```python
from build123d import *

# Parameters (mm, degrees)
SKETCH_1_R          = 102
EXTRUDE_1_DEPTH     = 12
SKETCH_2_R          = 69
EXTRUDE_2_DEPTH     = 3
SKETCH_3_R          = 63.5
EXTRUDE_3_DEPTH     = 1
SKETCH_4_R          = 55
CUT_EXTRUDE_1_DEPTH = 146.134420452
CUT_EXTRUDE_START   = -8
SKETCH_5_R          = 82
SKETCH_5_R_2        = 69
CUT_EXTRUDE_2_DEPTH = 4
SKETCH_6_R          = 4
CUT_EXTRUDE_3_DEPTH = 8
SKETCH_7_R          = 5
CUT_EXTRUDE_4_DEPTH = 146.134420452
CHAMFER_1_SIZE      = 0.5


with BuildPart() as part:
    # 草图1 → 凸台-拉伸1 (new body)
    with BuildSketch(Plane.XY):
        Circle(SKETCH_1_R)
    extrude(amount=EXTRUDE_1_DEPTH)

    # 草图2 → 凸台-拉伸2 (add)
    with BuildSketch(Plane.XY.offset(12)):
        Circle(SKETCH_2_R)
    extrude(amount=EXTRUDE_2_DEPTH)

    # 草图3 → 凸台-拉伸3 (add)
    with BuildSketch(Plane.XY.offset(15)):
        Circle(SKETCH_3_R)
    extrude(amount=EXTRUDE_3_DEPTH)

    # 草图4 → 切除-拉伸1 (cut, through all)
    with BuildSketch(Plane.XY.offset(16)):
        Circle(SKETCH_4_R)
    extrude(amount=-CUT_EXTRUDE_1_DEPTH, mode=Mode.SUBTRACT)

    # 草图5 → 切除-拉伸2 (cut)
    with BuildSketch(Plane.XY.offset(16).offset(CUT_EXTRUDE_START)):
        Circle(SKETCH_5_R)
        Circle(SKETCH_5_R_2, mode=Mode.SUBTRACT)
    extrude(amount=CUT_EXTRUDE_2_DEPTH, mode=Mode.SUBTRACT)

    # 草图6 → 切除-拉伸3 (cut)
    with BuildSketch(Plane.XY):
        with Locations(Location((-51.265241636, 51.265241636, 0), (0, 0, 286.819656348))):
            Circle(SKETCH_6_R)
        with Locations(Location((51.265241636, 51.265241636, 0), (0, 0, 180))):
            Circle(SKETCH_6_R)
        with Locations(Location((51.265241636, -51.265241636, 0), (0, 0, 163.180343652))):
            Circle(SKETCH_6_R)
        with Locations(Location((-51.265241636, -51.265241636, 0), (0, 0, 180))):
            Circle(SKETCH_6_R)
    extrude(amount=CUT_EXTRUDE_3_DEPTH, mode=Mode.SUBTRACT)

    # 草图7 → 切除-拉伸4 (cut, through all)
    with BuildSketch(Plane(origin=(0, 0, 0), x_dir=(-1, 0, 0), z_dir=(0, 0, -1))):
        with Locations((-77.942286341, 45)):
            Circle(SKETCH_7_R)
        with Locations((0, 90)):
            Circle(SKETCH_7_R)
        with Locations((77.942286341, 45)):
            Circle(SKETCH_7_R)
        with Locations((77.942286341, -45)):
            Circle(SKETCH_7_R)
        with Locations((0, -90)):
            Circle(SKETCH_7_R)
        with Locations((-77.942286341, -45)):
            Circle(SKETCH_7_R)
    extrude(amount=-CUT_EXTRUDE_4_DEPTH, mode=Mode.SUBTRACT)

    # 倒角1
    chamfer_1_edges = [part.edges().sort_by_distance(p)[0] for p in [
        (-82, 0, 12),
        (-102, 0, 0),
        (-102, 0, 12),
        (-69, 0, 15),
    ]]
    chamfer(chamfer_1_edges, length=CHAMFER_1_SIZE)


solid = part.part
```
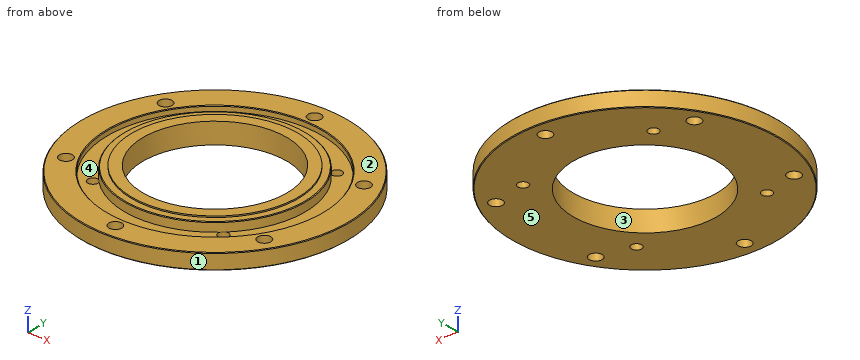
Build history of the part. All positions in model axes, mm. Face numbers are marked on the shaded views. A direction names the side the tool comes from. Give positions to 0.01 mm unless a question says otherwise; leave off trailing zeros. Order: outer loops, then holes, each group sorted by start corner. A loop starts at its lowest first (then second) coordinate and runs counter-clockwise, first axis right, second up. Notation, with made-up numbers: M 58.5,71 L 62.5,71 A19 ccw 62.5,90 Z; hole C -13.5,-10.75 d5. An arc over 180 degrees is marked long. Return JSON: item names as keys, results as strings.
Q1. Band-saw the part on A-A (y = 0). Give the cut face in (x, z).
Answer list:
{"outline": "M -102,0.5 L -101.5,0 L -55,0 L -55,16 L -63.5,16 L -63.5,15 L -68.5,15 L -69,14.5 L -69,8 L -82,8 L -82,11.5 L -82.5,12 L -101.5,12 L -102,11.5 Z; M 55,0 L 101.5,0 L 102,0.5 L 102,11.5 L 101.5,12 L 82.5,12 L 82,11.5 L 82,8 L 69,8 L 69,14.5 L 68.5,15 L 63.5,15 L 63.5,16 L 55,16 Z"}
Q2. Band-saw the part on B-B (z = 5.25). Count the separate pieces of the cut face and the enclosed holes in it, then the cut area to 3 significant figures.
Answer list:
{"separate pieces": "1", "enclosed holes": "11", "area": "22,500 mm^2"}
Q3. Flat gauge pins, fed straight in: pin 1 (4 mm diameter, centred on x = 74, z = 11, fed in from +Y); pin 2 (8 mm diameter, centred on x = 0, y = -90, fed in from -Z); pin 3 (1 mm diameter, centred on x = -30.5, z = 8, fed in from +Y); pin 4 (5 mm diameter, centred on y = 7.5, z = 8.5, fed in from -X). Where does each tip first touch, or does it go through?
Answer list:
{"pin 1": "stops at y = 72.25", "pin 2": "passes through", "pin 3": "stops at y = 97.49", "pin 4": "stops at x = -101.88"}
Q4. Wall check: probe 1 along Y at (x, z) = (0, 5); probe 2 along Y at (x, z) = (-56, 9.75); probe 3 along Y at (x, z) = (-25.5, 9). Give the ranges that are in metal, low to high. Write a range as from..to.
Answer list:
{"probe 1": "y = -102..-95, -85..-55, 55..85, 95..102", "probe 2": "y = -85.25..-59.9, -40.31..40.31, 59.9..85.25", "probe 3": "y = -98.76..-77.93, -64.12..-48.73, 48.73..64.12, 77.93..98.76"}
Q5. 3-axis set-ups, long thin cutter, end or side, ignore diameter. For the marked faces 4 and 5: which of +Z, -Z, +X, -X, +Y, -Y reach the whole face in a straight line?
Answer list:
{"face 4": "+Z", "face 5": "-Z, +X, -X, +Y, -Y"}
Q6. Two-plate mould, pull along Y, no slides. Class the marked faces 1, 2 and 3: pulls with the +Y half, pulls with the -Y half, needs draft (parallel to the pull), parting line crosses it, or undercut.
Answer list:
{"face 1": "parting line crosses it", "face 2": "needs draft", "face 3": "undercut"}
